Verification items for the finished model (mm, model axes). A direction names the side the tool comes from. Round coordinates to 2 decimals unless told otherwise and drop trailing zeros. Loops run counter-clockwise (first coordinate to the right, second up) from the corner with the lowest first, then second, coordinate; pieces in that order, holes last. Notation, with made-up numbers: (-39, 1.5) - (-29, 1.5) arc R18 cw to (-29, 5.5) - close; hole circle Ø6 at (34, 23.25). An arc over 180 degrees is marked (long way). Use CSV: the item, a comma, the result in double quotes.
```python
from build123d import *

# Parameters (mm, degrees)
BASE_FLANGE1_DEPTH = 3.175
SKETCH2_R          = 2.5781
SKETCH2_R_2        = 3.5687
SKETCH2_R_3        = 3.175
CUT_EXTRUDE1_DEPTH = 318.515874603
FILLET1_R          = 12.7
SKETCH3_R          = 82.55
CUT_EXTRUDE2_DEPTH = 318.515874603


# Sheet-metal steps are written as plain solids
with BuildPart() as part:
    # Sketch1 → Base-Flange1 (new body)
    with BuildSketch(Plane(origin=(0, 0, 0), x_dir=(1, 0, 0), z_dir=(0, 1, 0))):
        Polygon((152.4, -177.8), (-152.4, -177.8), (-152.4, 254), (152.4, 254), (152.4, -120.65), (190.5, -120.65), (190.5, -177.8), align=None)
    extrude(amount=-BASE_FLANGE1_DEPTH)

    # Sketch2 → Cut-Extrude1 (cut, through all)
    with BuildSketch(Plane(origin=(0, 0, 0), x_dir=(1, 0, 0), z_dir=(0, 1, 0))):
        with Locations(Location((-107.95, 0, 0), (0, 0, 270))):
            Circle(SKETCH2_R)
        with Locations(Location((0, 107.95, 0), (0, 0, 270))):
            Circle(SKETCH2_R)
        with Locations(Location((107.95, 0, 0), (0, 0, 270))):
            Circle(SKETCH2_R)
        with Locations(Location((85.03404521, 85.03404521, 0), (0, 0, 270))):
            Circle(SKETCH2_R_2)
        with Locations(Location((85.03404521, -85.03404521, 0), (0, 0, 270))):
            Circle(SKETCH2_R_2)
        with Locations(Location((0, -107.95, 0), (0, 0, 270))):
            Circle(SKETCH2_R)
        with Locations(Location((-85.03404521, -85.03404521, 0), (0, 0, 270))):
            Circle(SKETCH2_R_2)
        with Locations(Location((-85.03404521, 85.03404521, 0), (0, 0, 270))):
            Circle(SKETCH2_R_2)
        with Locations(Location((0, 241.3, 0), (0, 0, 270))):
            Circle(SKETCH2_R_3)
        with Locations(Location((-139.7, 241.3, 0), (0, 0, 270))):
            Circle(SKETCH2_R_3)
        with Locations(Location((0, -165.1, 0), (0, 0, 270))):
            Circle(SKETCH2_R_3)
        with Locations(Location((-139.7, -165.1, 0), (0, 0, 90))):
            Circle(SKETCH2_R_3)
        with Locations(Location((139.7, 241.3, 0), (0, 0, 90))):
            Circle(SKETCH2_R_3)
        with Locations(Location((177.8, -165.1, 0), (0, 0, 270))):
            Circle(SKETCH2_R_3)
        with Locations(Location((177.8, -133.35, 0), (0, 0, 270))):
            Circle(SKETCH2_R_3)
        with Locations(Location((114.3, -165.1, 0), (0, 0, 270))):
            Circle(SKETCH2_R_3)
        with Locations(Location((107.95, -79.375, 0), (0, 0, 270))):
            Circle(SKETCH2_R_3)
        with Locations(Location((114.3, -133.35, 0), (0, 0, 270))):
            Circle(SKETCH2_R_3)
        with Locations(Location((-107.95, -79.375, 0), (0, 0, 270))):
            Circle(SKETCH2_R_3)
        with Locations(Location((-107.95, -139.7, 0), (0, 0, 270))):
            Circle(SKETCH2_R_3)
    extrude(amount=-CUT_EXTRUDE1_DEPTH, mode=Mode.SUBTRACT)

    # Fillet1
    fillet1_edges = [part.edges().sort_by_distance(p)[0] for p in [
        (152.4, -1.5875, 120.65),
        (190.5, -1.5875, 120.65),
    ]]
    fillet(fillet1_edges, radius=FILLET1_R)

    # Sketch3 → Cut-Extrude2 (cut, through all)
    with BuildSketch(Plane(origin=(0, 0, 0), x_dir=(1, 0, 0), z_dir=(0, 1, 0))):
        with Locations(Location((0, 0, 0), (0, 0, 270))):
            Circle(SKETCH3_R)
        with BuildLine():
            Line((114.3, 203.2), (114.3, 133.198723718))
            ThreePointArc((114.3, 133.198723718), (110.682604916, 127.466763288), (103.951851852, 128.265437654))
            ThreePointArc((103.951851852, 128.265437654), (68.871193184, 150.049221089), (29.482142857, 162.44633961))
            ThreePointArc((29.482142857, 162.44633961), (22.000851686, 166.803163593), (19.05, 174.942211887))
            Line((19.05, 174.942211887), (19.05, 203.2))
            ThreePointArc((19.05, 203.2), (22.769743879, 212.180256121), (31.75, 215.9))
            Line((31.75, 215.9), (101.6, 215.9))
            ThreePointArc((101.6, 215.9), (110.580256121, 212.180256121), (114.3, 203.2))
        make_face()
        with BuildLine():
            Line((-101.6, 215.9), (-31.75, 215.9))
            ThreePointArc((-31.75, 215.9), (-22.769743879, 212.180256121), (-19.05, 203.2))
            Line((-19.05, 203.2), (-19.05, 174.942211887))
            ThreePointArc((-19.05, 174.942211887), (-22.000851686, 166.803163593), (-29.482142857, 162.44633961))
            ThreePointArc((-29.482142857, 162.44633961), (-68.871193184, 150.049221089), (-103.951851852, 128.265437654))
            ThreePointArc((-103.951851852, 128.265437654), (-110.682604916, 127.466763288), (-114.3, 133.198723718))
            Line((-114.3, 133.198723718), (-114.3, 203.2))
            ThreePointArc((-114.3, 203.2), (-110.580256121, 212.180256121), (-101.6, 215.9))
        make_face()
    extrude(amount=-CUT_EXTRUDE2_DEPTH, mode=Mode.SUBTRACT)


solid = part.part
```
1) Cross-section at B-B, the plane z = -12. Record the cut outline in (x, y) (3 decimals).
Returned:
outline,"(-152.4, -3.175) - (-81.673, -3.175) - (-81.673, 0) - (-152.4, 0) - close; (81.673, -3.175) - (152.4, -3.175) - (152.4, 0) - (81.673, 0) - close"
2) Cross-section at D-D, the plane y = -2.55. Count the separate pieces of the cut face and the enclosed holes in it, then the cut area to 3 significant figures.
Returned:
separate pieces,"1"
enclosed holes,"23"
area,"99,100 mm²"
3) Mould release check, pull along Z, two halves, no side actions. Record for faces 1 (the face through (156.22, -1.61, 117.03)), 2 (the face through (22.67, -1.57, -212.08)), 3 (the face through (21, 0, -89)): +Z half, -Z half, draft (parallel to the pull), parting line (faces both ways), or undercut.
Returned:
face 1,"-Z half"
face 2,"undercut"
face 3,"draft"
4) Gauge pin test, flat ends, axial feed: pin 1 Ø4 at (x, z) = (114.3, 133.35) entering from +Y; pin 2 Ø1.6 at (y, z) = (-2, -194.5) entering from +X. Record the tip position at first contact, or that the pin passes through.
Returned:
pin 1,"passes through"
pin 2,"stops at x = 152.4"
5) Thickness scan on probe 1 along X at (y, z) = (-0.8, 165.1) (3 decimals); probe 2 along Z at (x, y) = (177.8, -1.2) (3 decimals); probe 3 along Z at (x, y) = (-139.7, -1.55) (3 decimals). Record the ranges inside material, lowest first. Write a range as [from, to].
Returned:
probe 1,"x = [-152.4, -142.875], [-136.525, -3.175], [3.175, 111.125], [117.475, 174.625], [180.975, 190.5]"
probe 2,"z = [120.65, 130.175], [136.525, 161.925], [168.275, 177.8]"
probe 3,"z = [-254, -244.475], [-238.125, 161.925], [168.275, 177.8]"
6) Cross-section at A-A, the plane x = -25. Record the cut outline in (y, z) (3 decimals), then the cut area to 3 significant figures.
Returned:
outline,"(-3.175, -254) - (0, -254) - (0, -213.958) - (-3.175, -213.958) - close; (-3.175, -164.185) - (0, -164.185) - (0, -78.673) - (-3.175, -78.673) - close; (-3.175, 78.673) - (0, 78.673) - (0, 177.8) - (-3.175, 177.8) - close"
area,"713 mm²"
7) Cross-section at C-C, the plane x = 95. Record the cut outline in (y, z) (3 decimals).
Returned:
outline,"(-3.175, -254) - (0, -254) - (0, -215.9) - (-3.175, -215.9) - close; (-3.175, -135.03) - (0, -135.03) - (0, 177.8) - (-3.175, 177.8) - close"
8) Access from +Z, -Z, +X, -X, +Y, -Y to the whole of each face (thin tool, end or side, straight path). Record for faces 4 (the face through (186.88, -1.61, 124.47)), 5 (the face through (-68.34, -1.57, -150.29)).
Returned:
face 4,"-Z, +X, +Y, -Y"
face 5,"+Y, -Y"
